Read the model definition and answer for the solid it produces. Units are mm, in the model's axes. Face numbers are marked on the shaded views. A direction names the side the tool comes from. Round coordinates to 2 decimals unless told otherwise and drop trailing zeros. Loops run counter-clockwise (first coordinate to the right, second up) from the corner with the lowest first, then second, coordinate; pieces in that order, holes last. Notation, with made-up numbers: (74.5, 17.25) -> (120.5, 17.25) arc R7 ccw to (120.5, 23.25) -> close; hole circle Ø3 at (-24.5, 17.5). An arc over 180 degrees is marked (long way). Put each result on its own line as item: value.
Autodesk Inventor part; units mm, degrees
ref_plane "Work Plane1" through (7, 0, 0) normal (1, 0, 0) x (0, 1, 0)
ref_plane "XZ Plane" through (0, 0, 0) normal (0, 1, 0) x (-1, 0, 0)
ref_plane "XY Plane" through (0, 0, 0) normal (0, 0, 1) x (1, 0, 0)
ref_plane "Work Plane1" through (7, 0, 0) normal (1, 0, 0) x (0, 1, 0)
sketch "Sketch1" plane through (0, 0, 0) normal (0, 1, 0) x (-1, 0, 0)
  line L0 (0, 0) -> (-10, 0)
  line L1 (0, 0) -> (0, -10)
  line L2 (-10, 0) -> (-10, -5)
  line L3 (-10, -5) -> (0, -10)
  dimension "d0" = 10
  dimension "d1" = 10
  dimension "d2" = 5
revolve "Revolution1" add sketch "Sketch1" angle 360 about axis through (0, 0, 0) along (1, 0, 0)
sketch "Sketch2" plane through (7, 0, 0) normal (1, 0, 0) x (0, 1, 0)
  circle A0 centre (0, 0) radius 2.25
  dimension "d5" = 4.5
extrude "Extrusion1" cut sketch "Sketch2" along normal blind 2 and the other way blind 10
sketch "Sketch3" plane through (7, 0, 0) normal (1, 0, 0) x (0, 1, 0)
  line L0 (0, 0) -> (3.75, 0)
  line L1 (3.75, -2.1651) -> (0, -4.3301)
  line L2 (0, -4.3301) -> (-3.75, -2.1651)
  line L3 (-3.75, -2.1651) -> (-3.75, 2.1651)
  line L4 (-3.75, 2.1651) -> (0, 4.3301)
  line L5 (0, 4.3301) -> (3.75, 2.1651)
  line L6 (3.75, 2.1651) -> (3.75, -2.1651)
  line L7 (-3.75, 14.6203) -> (-3.75, 2.1651)
  line L8 (-3.75, 14.6203) -> (3.75, 14.6203)
  line L9 (3.75, 14.6203) -> (3.75, 1.2022)
  line L10 (3.75, 1.2022) -> (-3.75, 1.2022)
  line L11 (-3.75, 1.2022) -> (-3.75, 14.6203)
  dimension "d15" = 3.75
extrude "Extrusion2" cut sketch "Sketch3" against normal blind 4
sketch "Sketch5" plane through (9, 0, 0) normal (-1, 0, 0) x (0, 0, 1)
  circle A0 centre (0, 0) radius 2.25
extrude "Extrusion3" add sketch "Sketch5" along normal up to surface (2 mm away)
properties part number "stollen_m4"
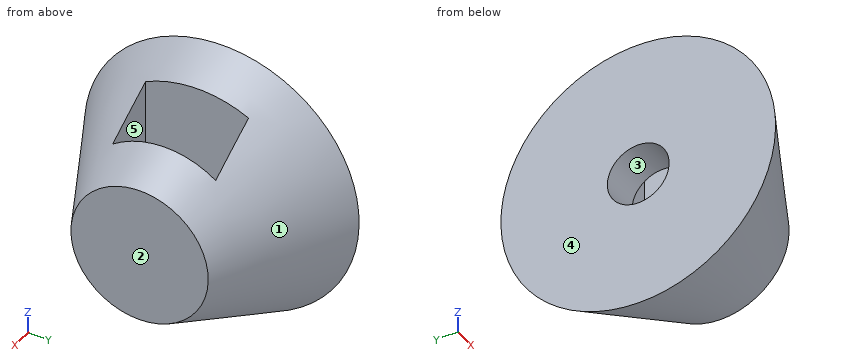
Item 1: The part is cut by section B-B (x = 8). Determine the outline of the cut face in (y, z), then the cut area to 3 significant figures.
Derived:
outline: circle Ø12 at (0, 0)
area: 113 mm^2
Item 2: Find the intervals of material crossed by line 1 along X through (y, z) = (2.5, -0.5); line 2 along X through (y, z) = (0.5, 6); line 3 along Y through (x, z) = (3.5, -4.25), in increasing order.
Derived:
line 1: x = 0 to 3, 7 to 10
line 2: x = 0 to 3, 7 to 7.96
line 3: y = -7.07 to -0.14, 0.14 to 7.07
Item 3: Which of the six approach directions +Z, -Z, +X, -X, +Y, -Y give full straight-line access (tool end or side, diameter ignored) to the marked faces 4 and 5?
Derived:
face 4: +Z, -Z, -X, +Y, -Y
face 5: +Z
Item 4: The part is cut by section C-C (x = 5). Determine the outline of the cut face in (y, z), then the cut area to 3 significant figures.
Derived:
outline: (-3.75, -2.17) -> (-3.75, 6.5) arc R7.5 ccw (long way) to (3.75, 6.5) -> (3.75, -2.17) -> (0, -4.33) -> close
area: 98.5 mm^2
Item 5: For a pull along Y with two mould halves and no side action, classify the marked faces 1, 2 and 3 as pulls with the +Y half, pulls with the -Y half, needs draft (parallel to the pull), parting line crosses it, or undercut.
Derived:
face 1: parting line crosses it
face 2: needs draft
face 3: undercut
Item 6: The part is cut by section A-A (z = 0). Determine the outline of the cut face in (x, y), then the cut area to 4 significant figures.
Derived:
outline: (0, -10) -> (10, -5) -> (10, 5) -> (0, 10) -> (0, 2.25) -> (3, 2.25) -> (3, 3.75) -> (7, 3.75) -> (7, -3.75) -> (3, -3.75) -> (3, -2.25) -> (0, -2.25) -> close
area: 106.5 mm^2
Item 7: Flat-ended cylindrical pins translate along their axes: pin 1 Ø3 at (x, z) = (6.5, -1.5) entering from -Y; pin 2 Ø1.5 at (x, z) = (1.5, -7.5) entering from -Y; pin 3 Ø3 at (x, z) = (4, 2.5) entering from -Y. Find the tip coordinate at first contact, or state that the pin passes through.
Derived:
pin 1: stops at y = -7.39
pin 2: stops at y = -6.49
pin 3: stops at y = -8.48
